Read the model definition and answer for the solid it produces. Units are mm, in the model's axes. A direction names the side the tool comes from. Coordinates: 2 decimals unless noted, no trailing zeros. Loops run counter-clockwise (first coordinate to the right, second up) from the corner with the lowest first, then second, coordinate; pieces in that order, holes last.
from build123d import *

# Parameters (mm, degrees)
F0_R      = 25.4
F1_DEPTH  = 152.4
F2_W      = 12.7
F2_H      = 76.2
F3_DEPTH  = 25.4
F4_W      = 12.7
F4_H      = 76.2
F5_DEPTH  = 38.1
F5_FACE_W = 6.35
F5_FACE_H = 76.2
F6_DEPTH  = 6.35


with BuildPart() as f1:
    # F0 (on Top) → F1 (new body)
    with BuildSketch(Plane.XY):
        Circle(F0_R)
    extrude(amount=F1_DEPTH)

    # F2 (on Right) → F3 (cut)
    with BuildSketch(Plane.YZ):
        with Locations((0, 76.2)):
            Rectangle(F2_W, F2_H)
    extrude(amount=-F3_DEPTH, mode=Mode.SUBTRACT)

    # F4 (on Front) → F5 (cut)
    with BuildSketch(Plane.XZ):
        with Locations((0, 76.2)):
            Rectangle(F4_W, F4_H)
    extrude(amount=F5_DEPTH, mode=Mode.SUBTRACT)

    # F5_face (on face) → F6 (cut)
    with BuildSketch(Plane(origin=(3.175, 0, 76.2), x_dir=(1, 0, 0), z_dir=(0, -1, 0))):
        Rectangle(F5_FACE_W, F5_FACE_H)
    extrude(amount=-F6_DEPTH, mode=Mode.SUBTRACT)


solid = f1.part
Item 1: Determine the mould class of faces 5 (the face through (0, 0, 0)), 6 (the face through (-6, -6, 38.1)), 7 (the face through (-9, 6.35, 76)), 8 (the face through (0, 0, 152.4)) for opening direction Z: released by +Z, released by -Z, zero draft, split by the parting line, or undercut.
Numbers:
face 5: released by -Z
face 6: undercut
face 7: undercut
face 8: released by +Z
Item 2: Find the intervals of material crossed by line 1 along Z through (x, y) = (-8.5, -4); line 2 along X through (y, z) = (-22.5, 71.5); line 3 along Y through (x, z) = (0.5, 87), in increasing order.
Numbers:
line 1: z = 0 to 38.1, 114.3 to 152.4
line 2: x = -11.79 to -6.35, 6.35 to 11.79
line 3: y = 6.35 to 25.4
Item 3: Given pin 1 (3 mm diameter, centred on x = -7.5, z = 50, fed in from -Y); pin 2 (9.5 mm diameter, centred on y = -15.5, z = 85, fed in from -X); pin 3 (10 mm diameter, centred on x = -3.5, z = 30, fed in from -Y), each flat-ended and moving along its own axis, determine where each tip first touches the part or whether it passes through.
Numbers:
pin 1: stops at y = -24.59
pin 2: stops at x = -23.01
pin 3: stops at y = -25.4
Item 4: A cutting plane is placed at A-A on y = 0. Determine the outline of the cut face in (x, z).
Numbers:
outline: (-25.4, 0) - (25.4, 0) - (25.4, 152.4) - (-25.4, 152.4) - (-25.4, 114.3) - (6.35, 114.3) - (6.35, 38.1) - (-25.4, 38.1) - close
Item 5: A cutting plane is placed at C-C on z = 45.5. Determine the outline of the cut face in (x, y), then the cut area to 3 significant figures.
Numbers:
outline: (-24.59, -6.35) arc R25.4 ccw to (-6.35, -24.59) - (-6.35, -6.35) - close; (-24.59, 6.35) - (6.35, 6.35) - (6.35, -24.59) arc R25.4 ccw (long way) to start
area: 1,390 mm2
Item 6: A cutting plane is placed at B-B on x = -21. Determine the outline of the cut face in (y, z).
Numbers:
outline: (-14.29, 0) - (14.29, 0) - (14.29, 152.4) - (-14.29, 152.4) - close; hole (-6.35, 38.1) - (6.35, 38.1) - (6.35, 114.3) - (-6.35, 114.3) - close
Item 7: Which of the six approach directions +Z, -Z, +X, -X, +Y, -Y give full straight-line access (tool end or side, diameter ignored) to faces 1 (the face through (-15, -6.35, 76)), 2 (the face through (-6, -6, 114.3)), 3 (the face through (-6.35, -15, 76)), 4 (the face through (24.227, 7.629, 75.133))?
Numbers:
face 1: -X
face 2: none
face 3: -Y
face 4: +Z, -Z
